from build123d import *

# Parameters (mm, degrees)
SKETCH1_W           = 370
SKETCH1_H           = 90
BOSS_EXTRUDE1_DEPTH = 5
SKETCH2_R           = 6.5
CUT_EXTRUDE1_DEPTH  = 10


with BuildPart() as part:
    # Sketch1 → Boss-Extrude1 (new body)
    with BuildSketch(Plane.XY):
        Rectangle(SKETCH1_W, SKETCH1_H)
    extrude(amount=BOSS_EXTRUDE1_DEPTH)

    # Sketch2 → Cut-Extrude1 (cut)
    with BuildSketch(Plane.XY.offset(5)):
        with Locations((150, -27.5)):
            Circle(SKETCH2_R)
        with Locations((-150, -27.5)):
            Circle(SKETCH2_R)
    extrude(amount=-CUT_EXTRUDE1_DEPTH, mode=Mode.SUBTRACT)


solid = part.part
Work out the finished part from the listing and answer in its coordinate system (mm). Round coordinates to 2 decimals unless told otherwise and drop trailing zeros. Write each loop counter-clockwise with the first axis right and the second up, starting at its lowest first coordinate (ties: lowest second). Pieces come first, ordered by that corner, then holes. Notation, with made-up numbers: M 22.25,23 L 67.25,23 A31 ccw 67.25,59 Z; hole C 7,68 d8. An arc over 180 degrees is marked long. Use a Markdown table: item, result.
1) Determine the mould class of faces 1 (the face through (-3, 1, 0)), 2 (the face through (143.506, -27.214, 2.535)), 3 (the face through (-156.494, -27.214, 2.535)) for opening direction X: pulls with the +X half, pulls with the -X half, needs draft (parallel to the pull), parting line crosses it, or undercut.
Taken from the geometry:
| item | result |
|---|---|
| face 1 | needs draft |
| face 2 | undercut |
| face 3 | undercut |
2) Consider line 1 (Y direction, x = 150, z = 3.35). Determine where the line is inside the solid, lowest interval first. Write a range as [from, to].
Taken from the geometry:
| item | result |
|---|---|
| line 1 | y = [-45, -34], [-21, 45] |
3) The part is cut by section A-A on x = 150. Give the vertices of the cut face in (y, z), plus the area to 3 significant figures.
Taken from the geometry:
| item | result |
|---|---|
| outline | M -45,0 L -34,0 L -34,5 L -45,5 Z; M -21,0 L 45,0 L 45,5 L -21,5 Z |
| area | 385 mm2 |
4) The part is cut by section B-B on y = -27.5. Give the vertices of the cut face in (x, z).
Taken from the geometry:
| item | result |
|---|---|
| outline | M -185,0 L -156.5,0 L -156.5,5 L -185,5 Z; M -143.5,0 L 143.5,0 L 143.5,5 L -143.5,5 Z; M 156.5,0 L 185,0 L 185,5 L 156.5,5 Z |
